Model file for the job. Use its own axes, mm. A direction names the side the tool comes from. Round coordinates to 2 decimals unless told otherwise and drop trailing zeros. Order: outer loops, then holes, each group sorted by start corner. A loop starts at its lowest first (then second) coordinate and runs counter-clockwise, first axis right, second up. Notation, with made-up numbers: (50, -31.5) - (61, -31.5) arc R12 ccw to (61, -11.5) - close; hole circle Ø5 at (20, 40). An arc over 180 degrees is marked (long way). Use one line per item in the form item = value.
from build123d import *

# Parameters (mm, degrees)
BASE_FLANGE1_DEPTH           = 3.175
M6_CLEARANCE_HOLE1_D         = 6.6
EDGE_FLANGE1_DEPTH           = 16.378
EDGE_FLANGE2_STRIP_W         = 14.1732
EDGE_FLANGE2_STRIP_H         = 3.175
EDGE_FLANGE2_STRIP_CUT_DEPTH = 16.378
EDGE_FLANGE2_DEPTH           = 16.378
M5_CLEARANCE_HOLE1_D         = 5.5
FILLET1_R                    = 2.54
FILLET2_R                    = 6.35


# Sheet-metal steps are written as plain solids
with BuildPart() as part:
    # Sketch1 → Base-Flange1 (new body)
    with BuildSketch(Plane.XY):
        Polygon((52.8905, -45.562600001), (36.5125, -45.562600001), (36.5125, -29.184600001), (61.9125, -29.184600001), (61.9125, -45.562600001), align=None)
    extrude(amount=-BASE_FLANGE1_DEPTH)

    # M6 Clearance Hole1 (through all)
    with Locations(Plane.XY):
        with Locations((46.0375, -37.373600001)):
            Hole(M6_CLEARANCE_HOLE1_D / 2)

    # Edge-Flange1 section (across the edge) → Edge-Flange1 (add)
    with BuildSketch(Plane(origin=(62.6491, -45.562600001, 0), x_dir=(-1, 0, 0), z_dir=(0, 1, 0))):
        with BuildLine():
            Line((-3.175, 0.7366), (-3.175, 23.9268))
            Line((-3.175, 23.9268), (0, 23.9268))
            Line((0, 23.9268), (0, 0.7366))
            ThreePointArc((0, 0.7366), (0.215745145, 0.215745145), (0.7366, 0))
            Line((0.7366, 0), (0.7366, -3.175))
            ThreePointArc((0.7366, -3.175), (-2.029318885, -2.029318885), (-3.175, 0.7366))
        make_face()
    extrude(amount=EDGE_FLANGE1_DEPTH)

    # Edge-Flange2 strip (across the edge) → Edge-Flange2 strip cut (cut)
    with BuildSketch(Plane(origin=(65.8241, -29.184600001, 23.9268), x_dir=(0, 0, -1), z_dir=(0, -1, 0))):
        with Locations((-6.35, -1.5875)):
            Rectangle(EDGE_FLANGE2_STRIP_W, EDGE_FLANGE2_STRIP_H)
    extrude(amount=EDGE_FLANGE2_STRIP_CUT_DEPTH, mode=Mode.SUBTRACT)

    # Edge-Flange2 section (across the edge) → Edge-Flange2 (add)
    with BuildSketch(Plane(origin=(65.8241, -29.184600001, 23.9268), x_dir=(0, 0, -1), z_dir=(0, -1, 0))):
        with BuildLine():
            Line((-3.175, 0.7366), (-3.175, 34.925))
            Line((-3.175, 34.925), (0, 34.925))
            Line((0, 34.925), (0, 0.7366))
            ThreePointArc((0, 0.7366), (0.215745145, 0.215745145), (0.7366, 0))
            Line((0.7366, 0), (0.7366, -3.175))
            ThreePointArc((0.7366, -3.175), (-2.029318885, -2.029318885), (-3.175, 0.7366))
        make_face()
    extrude(amount=EDGE_FLANGE2_DEPTH)

    # M5 Clearance Hole1 (through all)
    with Locations(Plane.XY.offset(27.1018)):
        with Locations((94.5499, -37.373600001)):
            Hole(M5_CLEARANCE_HOLE1_D / 2)

    # Fillet1
    fillet1_edges = [part.edges().sort_by_distance(p)[0] for p in [
        (100.7491, -29.184600001, 25.5143),
        (36.5125, -45.562600001, -1.5875),
        (36.5125, -29.184600001, -1.5875),
    ]]
    fillet(fillet1_edges, radius=FILLET1_R)

    # Fillet2
    fillet2_edges = [part.edges().sort_by_distance(p)[0] for p in [
        (100.7491, -45.562600001, 25.5143),
    ]]
    fillet(fillet2_edges, radius=FILLET2_R)


solid = part.part
(1) Slice it at B-B on x = 44.5. Give the cut face in (y, z) (3 decimals), then the cut area to 3 significant figures.
Report:
outline = (-45.563, -3.175) - (-40.294, -3.175) - (-40.294, 0) - (-45.563, 0) - close; (-34.454, -3.175) - (-29.185, -3.175) - (-29.185, 0) - (-34.454, 0) - close
area = 33.5 mm2
(2) Pull direction Y, two halves, no side cores. Call faces 1 (the face through (99.985, -29.909, 25.492)), 2 (the face through (49.334, -37.229, -1.61)), 3 (the face through (37.28, -44.84, -1.61)): released by +Y, released by -Y, zero draft, split by the parting line, or undercut.
Report:
face_1 = released by +Y
face_2 = undercut
face_3 = released by -Y
(3) Slice it at A-A on y = -35.75. Give the cut face in (x, z) (1 decimal), then the cut area to 3 significant figures.
Report:
outline = (36.5, -3.2) - (43.2, -3.2) - (43.2, 0) - (36.5, 0) - close; (48.9, -3.2) - (61.9, -3.2) arc R3.9 ccw to (65.8, 0.7) - (65.8, 23.2) arc R0.7 cw to (66.6, 23.9) - (92.3, 23.9) - (92.3, 27.1) - (66.6, 27.1) arc R3.9 ccw to (62.6, 23.2) - (62.6, 0.7) arc R0.7 cw to (61.9, 0) - (48.9, 0) - close; (96.8, 23.9) - (100.7, 23.9) - (100.7, 27.1) - (96.8, 27.1) - close
area = 251 mm2
(4) Tool access for faces 4 (the face through (84, -37, 23.927)), 5 (the face through (83, -37, 27.102)), 6 (the face through (49, -35, 0)): list every direction of +Z, -Z, +X, -X, +Y, -Y with a clear straight run to the whole face (end or side of a thin tool).
Report:
face_4 = -Z, +X, +Y, -Y
face_5 = +Z, +X, -X, +Y, -Y
face_6 = +Z, -X, +Y, -Y
(5) Slice it at C-C on y = -32.5. Give the cut face in (x, z) (1 decimal), then the cut area to 3 significant figures.
Report:
outline = (36.5, -3.2) - (61.9, -3.2) arc R3.9 ccw to (65.8, 0.7) - (65.8, 23.2) arc R0.7 cw to (66.6, 23.9) - (100.7, 23.9) - (100.7, 27.1) - (66.6, 27.1) arc R3.9 ccw to (62.6, 23.2) - (62.6, 0.7) arc R0.7 cw to (61.9, 0) - (36.5, 0) - close
area = 284 mm2
(6) Slice it at D-D on z = 4. Give the cut face in (x, y), then the cut area to 3 significant figures.
Report:
outline = (62.65, -45.56) - (65.82, -45.56) - (65.82, -29.18) - (62.65, -29.18) - close
area = 52.0 mm2
(7) Pin check, flat tips, straight feed: pin 1 (1.5 mm diameter, centred on x = 52.5, y = -36.5, fed in from +Z); pin 2 (8 mm diameter, centred on x = 60, z = 7, fed in from -Y); pin 3 (6 mm diameter, centred on x = 90, y = -33.5, fed in from -Z); pin 4 (6 mm diameter, centred on y = -31.5, z = 3.5, fed in from +X). Stop position of each tip, or through.
Report:
pin_1 = 0
pin_2 = -45.56
pin_3 = 23.93
pin_4 = 65.82
(8) Probe probe 1 along Z at (x, y) = (77, -36); probe 2 along X at (y, z) = (-39.5, 4); probe 3 along Z at (x, y) = (61, -36) (3 decimals). List the from-to ranges inside material, lowest first. Write a range as [from, to].
Report:
probe_1 = [23.93, 27.1]
probe_2 = [62.65, 65.82]
probe_3 = [-3.175, 0]
